Geometry check sheet. Reference: the model listing, model coordinates, mm. A direction names the side the tool comes from. Round coordinates to 2 decimals unless told otherwise and drop trailing zeros. Order: outer loops, then holes, each group sorted by start corner. A loop starts at its lowest first (then second) coordinate and runs counter-clockwise, first axis right, second up.
(1) Cross-section at D-D on z = 3.75. Enter the section's corners in (x, y).
(2) Cross-section at B-B on y = 1.5. Enter the section's corners in (x, z) (3 decimals).
(3) Thickness scan on L1, parallel to Z at x = 0, y = -1.5; L2, parallel to X at y = 2, z = 9; L3, parallel to Z at x = 1.5, y = 1.5. Record the ranges inside material, lowest first.
(4) Gauge pin test, flat ends, axial feed: P1, Ø1.2, axis at y = 1.5, z = 7, coming from the +X side; P2, Ø2, axis at y = 2, z = 4.5, coming from the -X side; P3, Ø3, axis at x = 0, z = 9, coming from the +Y side; P4, Ø2.5, axis at x = -9, z = -1, coming from the +Y side. Record the tip position at first contact, or that the pin passes through.
(5) Cross-section at C-C on x = 2.5. Enter the section's corners in (y, z), and give its area (3 significant figures).
(6) Set-up check for faces 4 (the face through (0, 2, 3.25)), 5 (the face through (9, -0.25, 0)), 6 (the face through (0, -3.75, 0)): record each of +Z, -Z, +X, -X, +Y, -Y from which the full face is reachable in a straight line by a thin tool's end or side.
(7) Cross-section at A-A on x = 0. Enter the section's corners in (y, z), and give its area (4 significant figures).
(8) Draft check along X on faces 1 (the face through (-9, -0.25, 0)), 2 (the face through (3.125, 2, -4)), 3 (the face through (-7.5, 2, 0)). Enter one of: pulls with the +X half, pulls with the -X half, needs draft (parallel to the pull), parting line crosses it, or undercut.
from build123d import *

# Parameters (mm, degrees)
BOSS_EXTRUDE1_DEPTH        = 14.75
SKETCH3_W                  = 6.25
SKETCH3_H                  = 4
CUT_EXTRUDE1_DEPTH         = 15
F_3_7_3_7_DIAMETER_HOLE1_D = 3.7


with BuildPart() as part:
    # Sketch1 → Boss-Extrude1 (new, symmetric)
    with BuildSketch(Plane.XY):
        Polygon((-7.5, -0.25), (-7.5, 3.75), (7.5, 3.75), (7.5, -0.25), (10.5, -0.25), (10.5, -3.75), (-10.5, -3.75), (-10.5, -0.25), align=None)
    extrude(amount=BOSS_EXTRUDE1_DEPTH, both=True)

    # Sketch3 → Cut-Extrude1 (cut)
    with BuildSketch(Plane(origin=(0, 0, -11.75), x_dir=(-1, 0, 0), z_dir=(0, 0, -1))):
        with Locations((0, 1.75)):
            Rectangle(SKETCH3_W, SKETCH3_H)
    extrude(amount=-CUT_EXTRUDE1_DEPTH, mode=Mode.SUBTRACT)

    # Ø3.7 (3.7) Diameter Hole1 (through all)
    with Locations(Plane(origin=(0, 3.75, 0), x_dir=(1, 0, 0), z_dir=(0, 1, 0))):
        with Locations((0, -9)):
            Hole(F_3_7_3_7_DIAMETER_HOLE1_D / 2)


solid = part.part
Found:
1. outline: (-10.5, -3.75) - (10.5, -3.75) - (10.5, -0.25) - (7.5, -0.25) - (7.5, 3.75) - (-7.5, 3.75) - (-7.5, -0.25) - (-10.5, -0.25) - close
2. outline: (-7.5, -14.75) - (7.5, -14.75) - (7.5, 14.75) - (-7.5, 14.75) - close; hole (-3.125, -11.75) - (3.125, -11.75) - (3.125, 3.25) - (-3.125, 3.25) - close; hole circle Ø3.7 at (0, 9)
3. L1: z = -14.75 to 7.15, 10.85 to 14.75
3. L2: x = -7.5 to -1.85, 1.85 to 7.5
3. L3: z = -14.75 to -11.75, 3.25 to 7.92, 10.08 to 14.75
4. P1: stops at x = 7.5
4. P2: stops at x = -7.5
4. P3: passes through
4. P4: stops at y = -0.25
5. outline: (-3.75, -14.75) - (3.75, -14.75) - (3.75, -11.75) - (-0.25, -11.75) - (-0.25, 3.25) - (3.75, 3.25) - (3.75, 14.75) - (-3.75, 14.75) - close
5. area: 161 mm2
6. face 4: +Y
6. face 5: +Z, -Z, +X, +Y
6. face 6: +Z, -Z, +X, -X, -Y
7. outline: (-3.75, -14.75) - (3.75, -14.75) - (3.75, -11.75) - (-0.25, -11.75) - (-0.25, 3.25) - (3.75, 3.25) - (3.75, 7.15) - (-3.75, 7.15) - close; (-3.75, 10.85) - (3.75, 10.85) - (3.75, 14.75) - (-3.75, 14.75) - close
7. area: 133.5 mm2
8. face 1: needs draft
8. face 2: undercut
8. face 3: pulls with the -X half
